Check sheet for the modelled part. Datum: model origin and axes. Units: mm. Face numbers are marked on the shaded views. A direction names the side the tool comes from. Give positions to 0.01 mm unless a question says otherwise; leave off trailing zeros. Write each loop counter-clockwise with the first axis right and the second up, starting at its lowest first coordinate (ties: lowest second). Pieces come first, ordered by that corner, then holes. Notation, with made-up numbers: M 10,44.25 L 67,44.25 A11 ccw 67,59.25 Z; hole C 58,55.5 d9. An arc over 180 degrees is marked long. Write item = value, one per line. Start each with the question number.
1) Sectioned sample at B-B, the plane x = 8.5. Record the cut outline in (y, z).
2) Draft check along Z on the marked faces 6, 7 and 8. Enter one of: pulls with the +Z half, pulls with the -Z half, needs draft (parallel to the pull), parting line crosses it, or undercut.
3) Scan lines: L1, parallel to Y at x = 9, z = 38; L2, parallel to X at y = 1.75, z = 14; L3, parallel to Z at x = 6.5, y = 0.5. Record each from-to range of solid material in increasing order.
4) Set-up check for the marked faces 1, 2, 3, 4 and 5: record each of +Z, -Z, +X, -X, +Y, -Y from which the full face is reachable in a straight line by a thin tool's end or side.
5) Gauge pin test, flat ends, axial feed: pin 1 (6.5 mm diameter, centred on x = 2, z = 27, fed in from -Y); pin 2 (5.5 mm diameter, centred on y = -1, z = 30, fed in from -X); pin 3 (11 mm diameter, centred on x = 5, z = 31, fed in from +Y). Record the tip position at first contact, or that the pin passes through.
6) Sectioned sample at A-A, the plane z = 39.5. Record the cut outline in (x, y), then the cut area to 3 significant figures.
7) Sectioned sample at C-C, the plane x = 0. Record the cut outline in (y, z).
8) Sectioned sample at D-D, the plane y = 0. Record the cut outline in (x, z).
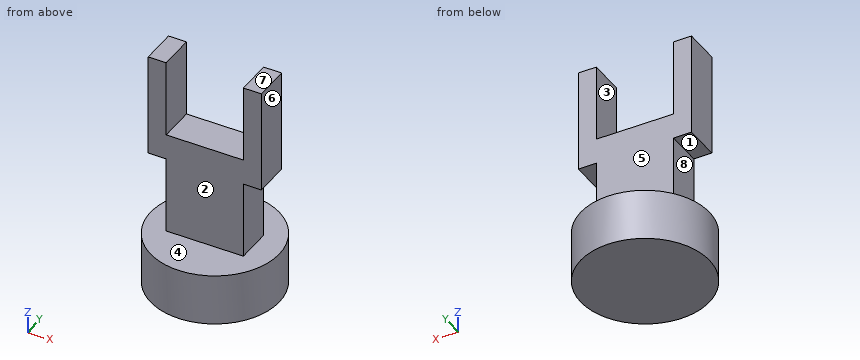
from build123d import *

# Parameters (mm, degrees)
SKETCH1_R             = 12.5
BOSS_EXTRUDE1_DEPTH   = 10
SKETCH2_W             = 15
SKETCH2_H             = 7
BOSS_EXTRUDE2_DEPTH   = 20
SKETCH3_W             = 3.5
SKETCH3_H             = 7
BOSS_EXTRUDE4_DEPTH   = 15
BOSS_EXTRUDE4_2_DEPTH = 15
SKETCH3_4_W           = 3.5
SKETCH3_4_H           = 7
BOSS_EXTRUDE5_DEPTH   = 5


with BuildPart() as part:
    # Sketch1 → Boss-Extrude1 (new body)
    with BuildSketch(Plane.XY):
        Circle(SKETCH1_R)
    extrude(amount=BOSS_EXTRUDE1_DEPTH)

    # Sketch2 → Boss-Extrude2 (add)
    with BuildSketch(Plane.XY.offset(10)):
        Rectangle(SKETCH2_W, SKETCH2_H)
    extrude(amount=BOSS_EXTRUDE2_DEPTH)



with BuildPart() as body_2:
    # Sketch3 → Boss-Extrude4 (new body)
    with BuildSketch(Plane.XY.offset(30)):
        with Locations((-9.25, 0)):
            Rectangle(SKETCH3_W, SKETCH3_H)
    extrude(amount=BOSS_EXTRUDE4_DEPTH)


with BuildPart() as body_3:
    # Sketch3 → Boss-Extrude4 2 (new body)
    with BuildSketch(Plane.XY.offset(30)):
        with Locations((9.25, 0)):
            Rectangle(SKETCH3_W, SKETCH3_H)
    extrude(amount=BOSS_EXTRUDE4_2_DEPTH)


with BuildPart() as part_1:
    add(part.part)

    add(body_2.part)  # Boss-Extrude5 merges body 2

    add(body_3.part)  # Boss-Extrude5 merges body 3
    # Sketch3<4> → Boss-Extrude5 (add)
    with BuildSketch(Plane.XY.offset(30)):
        with Locations((-9.25, 0)):
            Rectangle(SKETCH3_4_W, SKETCH3_4_H)
        with Locations((9.25, 0)):
            Rectangle(SKETCH3_4_W, SKETCH3_4_H)
    extrude(amount=-BOSS_EXTRUDE5_DEPTH)


solid = part_1.part
Data:
q1.outline = M -9.17,0 L 9.17,0 L 9.17,10 L -9.17,10 Z; M -3.5,25 L 3.5,25 L 3.5,45 L -3.5,45 Z
q2.face_6 = needs draft
q2.face_7 = pulls with the +Z half
q2.face_8 = undercut
q3.L1 = -3.5 to 3.5
q3.L2 = -7.5 to 7.5
q3.L3 = 0 to 30
q4.face_1 = -X, +Y, -Y
q4.face_2 = +Z, +X, -X, -Y
q4.face_3 = +Z, +Y, -Y
q4.face_4 = none
q4.face_5 = +Z, +X, -X, +Y
q5.pin_1 = -3.5
q5.pin_2 = -11
q5.pin_3 = 3.5
q6.outline = M -11,-3.5 L -7.5,-3.5 L -7.5,3.5 L -11,3.5 Z; M 7.5,-3.5 L 11,-3.5 L 11,3.5 L 7.5,3.5 Z
q6.area = 49.0 mm2
q7.outline = M -12.5,0 L 12.5,0 L 12.5,10 L 3.5,10 L 3.5,30 L -3.5,30 L -3.5,10 L -12.5,10 Z
q8.outline = M -12.5,0 L 12.5,0 L 12.5,10 L 7.5,10 L 7.5,25 L 11,25 L 11,45 L 7.5,45 L 7.5,30 L -7.5,30 L -7.5,45 L -11,45 L -11,25 L -7.5,25 L -7.5,10 L -12.5,10 Z
